Here's how the part is built. I have some questions about the finished solid (model axes, mm). Round coordinates to 2 decimals unless told otherwise and drop trailing zeros. Loops run counter-clockwise (first coordinate to the right, second up) from the corner with the lowest first, then second, coordinate; pieces in that order, holes last. Notation, with made-up numbers: M -22,55 L 18,55 A12 cw 18,67 Z; hole C -5,-25.75 d8. An arc over 180 degrees is marked long. One line per question, with ' | ' between items. Start each with the question number.
```python
from build123d import *

# Parameters (mm, degrees)
PAD_DEPTH = 1


with BuildPart() as part:
    # Sketch → Pad (new body)
    with BuildSketch(Plane.YZ.offset(-500)):
        with BuildLine():
            ThreePointArc((-427.08313, 260), (-481.76976, -133.783027), (-231.870564, -442.985374))
            ThreePointArc((-231.870564, -442.985374), (17.120198, -499.706813), (261.645072, -426.077289))
            ThreePointArc((261.645072, -426.077289), (430.453315, -254.381492), (499.438281, -23.693945))
            Line((499.438281, 340), (499.438281, -23.693945))
            Line((380, 340), (499.438281, 340))
            Line((380, 460), (380, 340))
            Line((230, 460), (380, 460))
            Line((230, 530), (230, 460))
            Line((0, 530), (230, 530))
            Line((0, 1040), (0, 530))
            Line((-658.874021, 1040), (0, 1040))
            Line((-658.874021, 1040), (-658.874021, 540))
            Line((-427.08313, 260), (-658.874021, 540))
        make_face()
    extrude(amount=-PAD_DEPTH)


solid = part.part
```
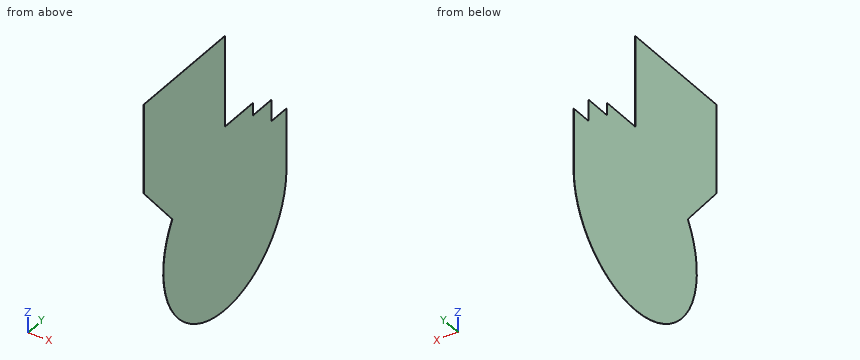
1) Imagine slicing it at B-B (y = -451.5). Write out the boundary of the cut face in (x, z).
2) Please list where these lines run through material, in increasing order: L1, parallel to Y at x = -500.25, z = 936; L2, parallel to Z at x = -500.45, y = -5 (3 decimals); L3, parallel to Z at x = -500.65, y = -220. Write a range as from..to.
3) I'm going to push flat-ended pins straight in: pin 1 Ø0.5 at (x, y) = (-500.5, 439.5) entering from +Z; pin 2 Ø0.5 at (x, z) = (-500.5, 658) entering from +Y. Where does each tip first touch, or does it pass through?
4) Imagine slicing it at C-C (z = 557.5). Write out the boundary of the cut face in (x, y).
5) Imagine slicing it at A-A (x = -500.25). Write out the boundary of the cut face in (y, z), then the cut area to 3 significant figures.
6) Imagine slicing it at D-D (y = 412.5). Write out the boundary of the cut face in (x, z), then the cut area to 3 significant figures.
Results are:
1) outline: M -501,-214.82 L -500,-214.82 L -500,214.82 L -501,214.82 Z; M -501,289.5 L -500,289.5 L -500,1040 L -501,1040 Z
2) L1: -658.87..0 | L2: -499.975..1040 | L3: -449..1040
3) pin 1: z = 340 | pin 2: y = 0
4) outline: M -501,-658.87 L -500,-658.87 L -500,0 L -501,0 Z
5) outline: M -658.87,540 L -427.08,260 A500 ccw -231.87,-442.99 A500 ccw 499.44,-23.69 L 499.44,340 L 380,340 L 380,460 L 230,460 L 230,530 L 0,530 L 0,1040 L -658.87,1040 Z | area: 1,230,000 mm²
6) outline: M -501,-282.57 L -500,-282.57 L -500,340 L -501,340 Z | area: 623 mm²
